The listing builds one solid part. Answer for the finished solid, in the listing's coordinates (mm). A direction names the side the tool comes from. Round coordinates to 2 decimals unless told otherwise and drop trailing zeros. Order: outer loops, then holes, each group sorted by start corner. A loop starts at its lowest first (then second) coordinate and runs counter-clockwise, first axis right, second up. Notation, with made-up numbers: (11, 25.5) -> (39, 25.5) arc R24 ccw to (39, 57.5) -> close; hole circle Ø5 at (72, 40.25). An arc over 180 degrees is marked (long way). Answer in a Markdown table with one row per item. Add a question column.
```python
from build123d import *

# Parameters (mm, degrees)
SKETCH2_R           = 1
SKETCH2_R_2         = 2
BOSS_EXTRUDE1_DEPTH = 5


with BuildPart() as part:
    # Sketch2 → Boss-Extrude1 (new body)
    with BuildSketch(Plane.XY):
        with BuildLine():
            Line((10.773856573, 0), (-10.773856573, 0))
            ThreePointArc((-10.773856573, 0), (-12.807539789, -0.432272712), (-14.489580701, -1.654346968))
            Line((-14.489580701, -1.654346968), (-32.85230533, -22.048218747))
            ThreePointArc((-32.85230533, -22.048218747), (-33.804483335, -23.602032031), (-34.136581202, -25.393871779))
            Line((-34.136581202, -25.393871779), (-34.136581202, -27.926924356))
            ThreePointArc((-34.136581202, -27.926924356), (-34.681548581, -30.196876855), (-36.197654941, -31.972009328))
            Line((-36.197654941, -31.972009328), (-47.938926261, -40.502542276))
            ThreePointArc((-47.938926261, -40.502542276), (-49.455032621, -42.277674749), (-50, -44.547627247))
            Line((-50, -44.547627247), (-50, -113.7061014))
            ThreePointArc((-50, -113.7061014), (-49.840547901, -114.95873703), (-49.372361591, -116.131478508))
            Line((-49.372361591, -116.131478508), (-38.744938669, -135.290122192))
            ThreePointArc((-38.744938669, -135.290122192), (-36.909614174, -137.173276478), (-34.372577077, -137.864745084))
            Line((-34.372577077, -137.864745084), (-29.364406032, -137.864745084))
            ThreePointArc((-29.364406032, -137.864745084), (-27.094453533, -138.409712463), (-25.31932106, -139.925818823))
            Line((-25.31932106, -139.925818823), (-19.497457724, -147.938926261))
            ThreePointArc((-19.497457724, -147.938926261), (-17.722325251, -149.455032621), (-15.452372753, -150))
            Line((-15.452372753, -150), (15.452372753, -150))
            ThreePointArc((15.452372753, -150), (17.722325251, -149.455032621), (19.497457724, -147.938926261))
            Line((19.497457724, -147.938926261), (25.31932106, -139.925818823))
            ThreePointArc((25.31932106, -139.925818823), (27.094453533, -138.409712463), (29.364406032, -137.864745084))
            Line((29.364406032, -137.864745084), (34.372577077, -137.864745084))
            ThreePointArc((34.372577077, -137.864745084), (36.909614174, -137.173276478), (38.744938669, -135.290122192))
            Line((38.744938669, -135.290122192), (49.372361591, -116.131478508))
            ThreePointArc((49.372361591, -116.131478508), (49.840547901, -114.95873703), (50, -113.7061014))
            Line((50, -113.7061014), (50, -44.547627247))
            ThreePointArc((50, -44.547627247), (49.455032621, -42.277674749), (47.938926261, -40.502542276))
            Line((47.938926261, -40.502542276), (36.197654941, -31.972009328))
            ThreePointArc((36.197654941, -31.972009328), (34.681548581, -30.196876855), (34.136581202, -27.926924356))
            Line((34.136581202, -27.926924356), (34.136581202, -25.393871779))
            ThreePointArc((34.136581202, -25.393871779), (33.804483335, -23.602032031), (32.85230533, -22.048218747))
            Line((32.85230533, -22.048218747), (14.489580701, -1.654346968))
            ThreePointArc((14.489580701, -1.654346968), (12.807539789, -0.432272712), (10.773856573, 0))
        make_face()
        with Locations((0, -5)):
            Circle(SKETCH2_R, mode=Mode.SUBTRACT)
        with Locations((0, -145)):
            Circle(SKETCH2_R_2, mode=Mode.SUBTRACT)
        with Locations((0, -105)):
            Circle(SKETCH2_R_2, mode=Mode.SUBTRACT)
        with Locations((-12, -50.308044585)):
            Circle(SKETCH2_R_2, mode=Mode.SUBTRACT)
        with Locations((12, -50.308044585)):
            Circle(SKETCH2_R_2, mode=Mode.SUBTRACT)
        with Locations((12, -85.308044585)):
            Circle(SKETCH2_R_2, mode=Mode.SUBTRACT)
        with Locations((-12, -85.308044585)):
            Circle(SKETCH2_R_2, mode=Mode.SUBTRACT)
        with Locations((-34.372577077, -132.864745084)):
            Circle(SKETCH2_R_2, mode=Mode.SUBTRACT)
        with Locations((34.372577077, -132.864745084)):
            Circle(SKETCH2_R_2, mode=Mode.SUBTRACT)
        with Locations((-45, -44.547627247)):
            Circle(SKETCH2_R_2, mode=Mode.SUBTRACT)
        with Locations((45, -44.547627247)):
            Circle(SKETCH2_R_2, mode=Mode.SUBTRACT)
        with BuildLine():
            Line((-12.660728973, -13.073490301), (-26.043341101, -27.93638681))
            ThreePointArc((-26.043341101, -27.93638681), (-28.867891964, -28.084415248), (-29.015920402, -25.259864385))
            Line((-29.015920402, -25.259864385), (-15.633308275, -10.396967875))
            ThreePointArc((-15.633308275, -10.396967875), (-12.808757412, -10.248939437), (-12.660728973, -13.073490301))
        make_face(mode=Mode.SUBTRACT)
        with BuildLine():
            Line((14.147018624, -37.43638681), (19.147018624, -37.43638681))
            ThreePointArc((19.147018624, -37.43638681), (20.458982346, -36.663539609), (20.41901608, -35.1413884))
            Line((20.41901608, -35.1413884), (15.41901608, -27.1413884))
            ThreePointArc((15.41901608, -27.1413884), (13.733494855, -26.494513691), (12.647018624, -27.93638681))
            Line((12.647018624, -27.93638681), (12.647018624, -35.93638681))
            ThreePointArc((12.647018624, -35.93638681), (13.086358453, -36.997046982), (14.147018624, -37.43638681))
        make_face(mode=Mode.SUBTRACT)
        with BuildLine():
            Line((-14.147018624, -37.43638681), (-19.147018624, -37.43638681))
            ThreePointArc((-19.147018624, -37.43638681), (-20.458982346, -36.663539609), (-20.41901608, -35.1413884))
            Line((-20.41901608, -35.1413884), (-15.41901608, -27.1413884))
            ThreePointArc((-15.41901608, -27.1413884), (-13.733494855, -26.494513691), (-12.647018624, -27.93638681))
            Line((-12.647018624, -27.93638681), (-12.647018624, -35.93638681))
            ThreePointArc((-12.647018624, -35.93638681), (-13.086358453, -36.997046982), (-14.147018624, -37.43638681))
        make_face(mode=Mode.SUBTRACT)
        with BuildLine():
            Line((12.660728973, -13.073490301), (26.043341101, -27.93638681))
            ThreePointArc((26.043341101, -27.93638681), (28.867891964, -28.084415248), (29.015920402, -25.259864385))
            Line((29.015920402, -25.259864385), (15.633308275, -10.396967875))
            ThreePointArc((15.633308275, -10.396967875), (12.808757412, -10.248939437), (12.660728973, -13.073490301))
        make_face(mode=Mode.SUBTRACT)
        with BuildLine():
            Line((1.5, -15), (1.5, -30))
            ThreePointArc((1.5, -30), (0, -31.5), (-1.5, -30))
            Line((-1.5, -30), (-1.5, -15))
            ThreePointArc((-1.5, -15), (0, -13.5), (1.5, -15))
        make_face(mode=Mode.SUBTRACT)
    extrude(amount=BOSS_EXTRUDE1_DEPTH)


solid = part.part
```
Item 1: For a pull along X with two mould halves and no side action, classify faces 4 (the face through (42.15, -36.297, 2.465)), 5 (the face through (-41.99, -36.18, 2.46)), 6 (the face through (-17.954, -31.197, 2.465)) as released by +X, released by -X, zero draft, split by the parting line, or undercut.
Item 2: Find the intervals of material crossed by probe 1 along Y at (x, z) = (0, 2.85); probe 2 along Y at (x, z) = (12.5, 0.9); probe 3 along X at (y, z) = (-131.5, 3.65), in increasing order. Write a range as [from, to].
Item 3: The part is cut by section A-A, the plane x = -45. Give the vertices of the cut face in (y, z), and give its area (3 significant figures).
Item 4: The part is cut by section C-C, the plane z = 1.55. State how many separate pieces and enclosed holes the cut face has, and give its area (3 significant figures).
Item 5: A tool of negligible diameter and unlimited length cuts with its end or side. For faces 1 (the face through (50, -80, 2)), 2 (the face through (13.76, -26.487, 2.465)), 3 (the face through (-32, -137.865, 2)), from which of +Z, -Z, +X, -X, +Y, -Y can it reach the whole face along a straight path? Write none if from no direction.
Item 6: The part is cut by section B-B, the plane y = -145. Give the vertices of the cut face in (x, z).
Item 7: Flat-ended cylindrical pins translate along their axes: P1, Ø3.5, axis at x = 12, y = -50.31, coming from the +Z side (3 decimals); P2, Ø1.5, axis at y = -24, z = 1.5, coming from the -X side; P3, Ø0.8, axis at y = -26, z = 2, coming from the +X side; P4, Ø1.5, axis at x = -16, z = 3.5, coming from the +Y side. Find the tip coordinate at first contact, or state that the pin passes through.
Resolved:
| question | item | result |
|---|---|---|
| 1 | face 4 | released by +X |
| 1 | face 5 | released by -X |
| 1 | face 6 | undercut |
| 2 | probe 1 | [-150, -147], [-143, -107], [-103, -31.5], [-13.5, -6], [-4, 0] |
| 2 | probe 2 | [-150, -87.24], [-83.37, -52.24], [-48.37, -12.87], [-10.6, -0.31] |
| 2 | probe 3 | [-40.85, -35.83], [-32.91, 32.91], [35.83, 40.85] |
| 3 | outline | (-124.01, 0) -> (-46.55, 0) -> (-46.55, 5) -> (-124.01, 5) -> close; (-42.55, 0) -> (-38.37, 0) -> (-38.37, 5) -> (-42.55, 5) -> close |
| 3 | area | 408 mm2 |
| 4 | separate pieces | 1 |
| 4 | enclosed holes | 16 |
| 4 | area | 11,900 mm2 |
| 5 | face 1 | +Z, -Z, +X, +Y, -Y |
| 5 | face 2 | +Z, -Z |
| 5 | face 3 | +Z, -Z, -X, -Y |
| 6 | outline | (-21.63, 0) -> (-2, 0) -> (-2, 5) -> (-21.63, 5) -> close; (2, 0) -> (21.63, 0) -> (21.63, 5) -> (2, 5) -> close |
| 7 | P1 | through |
| 7 | P2 | x = -34.09 |
| 7 | P3 | x = 34.14 |
| 7 | P4 | y = -2.5 |
